Autodesk Inventor part; units mm, degrees
ref_plane "YZ Plane" through (0, 0, 0) normal (1, 0, 0) x (0, 1, 0)
ref_plane "XZ Plane" through (0, 0, 0) normal (0, 1, 0) x (-1, 0, 0)
ref_plane "XY Plane" through (0, 0, 0) normal (0, 0, 1) x (1, 0, 0)
ref_plane "Work Plane2" through (35.545, -31.609, 1.6) normal (0, 0, 1) x (1, 0, 0)
ref_plane "Work Plane1" through (35.545, -31.609, 1.6) normal (0, 0, 1) x (1, 0, 0)
sketch "Sketch1" plane through (35.545, -31.609, 1.6) normal (0, 0, 1) x (1, 0, 0)
  line L0 (0, 0) -> (336, 0)
  line L1 (-2, -129) -> (-2, -2)
  line L2 (-1.6825, -0.9187) -> (-1.5115, -0.6903)
  arc A0 (0, 0) -> (-2, -2) centre (0, -2) ccw
  line L3 (338, -2) -> (338, -129)
  line L4 (337.5115, -0.6903) -> (337.6825, -0.9187)
  arc A1 (338, -2) -> (336, 0) centre (336, -2) ccw
  line L5 (336, -131) -> (0, -131)
  line L6 (337.6825, -130.0813) -> (337.5115, -130.3097)
  arc A2 (336, -131) -> (338, -129) centre (336, -129) ccw
  arc A3 (-2, -129) -> (0, -131) centre (0, -129) ccw
  circle A4 centre (1.98, -128.63) radius 1.1
  circle A5 centre (1.98, -128.63) radius 1.1
  circle A6 centre (68.313, -128.63) radius 1.1
  circle A7 centre (134.646, -128.63) radius 1.1
  circle A8 centre (134.646, -128.63) radius 1.1
  circle A9 centre (68.313, -128.63) radius 1.1
  circle A10 centre (200.979, -128.63) radius 1.1
  circle A11 centre (267.312, -128.63) radius 1.1
  circle A12 centre (333.645, -128.63) radius 1.1
  circle A13 centre (333.645, -128.63) radius 1.1
  circle A14 centre (267.312, -128.63) radius 1.1
  circle A15 centre (200.979, -128.63) radius 1.1
  circle A16 centre (333.638, -2.355) radius 1.1
  circle A17 centre (1.973, -2.355) radius 1.1
  circle A18 centre (68.306, -2.355) radius 1.1
  circle A19 centre (134.639, -2.355) radius 1.1
  circle A20 centre (200.972, -2.355) radius 1.1
  circle A21 centre (267.305, -2.355) radius 1.1
  circle A22 centre (333.645, -2.355) radius 1.093
  circle A23 centre (267.305, -2.355) radius 1.1
  circle A24 centre (200.972, -2.355) radius 1.1
  circle A25 centre (134.639, -2.355) radius 1.1
  circle A26 centre (68.306, -2.355) radius 1.1
  circle A27 centre (1.973, -2.355) radius 1.1
  line L7 (3, -4.2357) -> (125.2758, -4.2357) construction
  line L8 (4, -5) -> (332, -5)
  line L9 (333, -6) -> (333, -125)
  line L10 (332, -126) -> (4, -126)
  line L11 (3, -125) -> (3, -6)
  arc A28 (4, -5) -> (3, -6) centre (4, -6) ccw
  arc A29 (333, -6) -> (332, -5) centre (332, -6) ccw
  arc A30 (332, -126) -> (333, -125) centre (332, -125) ccw
  arc A31 (3, -125) -> (4, -126) centre (4, -125) ccw
  circle A32 centre (320.737, -95.692) radius 0.175
  line L12 (257.6125, -126) -> (315.0362, -126)
  line L13 (315.0362, -126) -> (315.0362, -126.7604)
  line L14 (315.0362, -126.7604) -> (257.6125, -126.7604)
  line L15 (257.6125, -126.7604) -> (257.6125, -126)
  point P0 (-35.545, 31.609)
  point P1 (-1.5115, -130.3097)
  point P2 (162.5077, 0)
  point P3 (162.5077, -5)
  point P4 (173.4174, -5)
  point P5 (173.4174, 0)
  point P6 (333, -88.192)
  point P7 (338, -88.192)
  point P8 (333, -102.192)
  point P9 (338, -102.192)
  point P10 (335.5, -88.192)
  point P11 (0, -131)
  point P12 (337.6825, -130.0813)
  point P13 (-1.6825, -0.9187)
  point P14 (337.6825, -0.9187)
  dimension "d2" = 5
  dimension "d3" = 5
  dimension "d4" = 5
  dimension "d5" = 5
  dimension "d6" = 1
  dimension "d7" = 1
  dimension "d8" = 1
  dimension "d9" = 1
extrude "Extrusion3" add sketch "Sketch1" along normal blind 3 contours L0 A1 L4 L3 A2 L6 L5 A3 L1 A0 L2
properties part number "top-layer"
Geometry: final body of the model. Coordinates: model frame, mm. Round coordinates to 2 decimals unless told otherwise and drop trailing zeros. Write each loop counter-clockwise with the first axis right and the second up, starting at its lowest first coordinate (ties: lowest second). Pieces come first, ordered by that corner, then holes. Notation, with made-up numbers: M -25.75,30 L 25.25,30 A25 ccw 25.25,44 Z; hole C 83.25,80.5 d4. An arc over 180 degrees is marked long. Answer in a Markdown table with one row per item. Add a question column.
(1) Cut plane A-A, the plane x = 197. Return the cut outline in (y, z), then the cut area to 3 significant figures.
(2) Ray query, L1, parallel to X at y = -107, z = 3.6 (3 decimals); L2, parallel to Y at x = 281, z = 1.9; L3, parallel to Y at x = 298, z = 1.8. Return the intervals inside material, ascending.
(3) Cut plane B-B, the plane y = -121.5. Return the cut outline in (x, z) (3 decimals), then the cut area to 3 significant figures.
(4) Cut plane C-C, the plane z = 3.1. Give the number of separate pieces and of enclosed holes in the cut face, then the cut area to 3 significant figures.
Established:
| question | item | result |
|---|---|---|
| 1 | outline | M -162.61,1.6 L -157.61,1.6 L -157.61,4.6 L -162.61,4.6 Z; M -36.61,1.6 L -31.61,1.6 L -31.61,4.6 L -36.61,4.6 Z |
| 1 | area | 30.0 mm² |
| 2 | L1 | 33.545 to 38.545, 368.545 to 373.545 |
| 2 | L2 | -162.61 to -157.61, -36.61 to -31.61 |
| 2 | L3 | -162.61 to -158.37, -36.61 to -31.61 |
| 3 | outline | M 33.545,1.6 L 38.545,1.6 L 38.545,4.6 L 33.545,4.6 Z; M 368.545,1.6 L 373.545,1.6 L 373.545,4.6 L 368.545,4.6 Z |
| 3 | area | 30.0 mm² |
| 4 | separate pieces | 1 |
| 4 | enclosed holes | 13 |
| 4 | area | 4,520 mm² |
